Autodesk Fusion 360 part; units mm, degrees
sketch "Sketch1" plane through (0, 0, 0) normal (0, 0, 1) x (1, 0, 0)
  line L0 (66, 26) -> (-66, 26)
  line L1 (-70, 22) -> (-70, -22)
  line L2 (-66, -26) -> (66, -26)
  line L3 (70, -22) -> (70, 22)
  line L4 (70, 26) -> (-70, -26) construction
  line L5 (-70, 26) -> (70, -26) construction
  arc A0 (-70, -22) -> (-66, -26) centre (-66, -22) ccw
  arc A1 (-66, 26) -> (-70, 22) centre (-66, 22) ccw
  arc A2 (70, 22) -> (66, 26) centre (66, 22) ccw
  arc A3 (66, -26) -> (70, -22) centre (66, -22) ccw
  line L6 (-70, 26) -> (-57, 26) construction
  line L7 (-57, 26) -> (-57, 12.5) construction
  line L8 (-57, 12.5) -> (-70, 12.5) construction
  line L9 (-70, 12.5) -> (-70, 26) construction
  line L10 (70, 26) -> (57, 26) construction
  line L11 (57, 26) -> (57, 12.5) construction
  line L12 (57, 12.5) -> (70, 12.5) construction
  line L13 (70, 12.5) -> (70, 26) construction
  line L14 (-70, -26) -> (-57, -26) construction
  line L15 (-57, -26) -> (-57, -12.5) construction
  line L16 (-57, -12.5) -> (-70, -12.5) construction
  line L17 (-70, -12.5) -> (-70, -26) construction
  line L18 (70, -26) -> (57, -26) construction
  line L19 (57, -26) -> (57, -12.5) construction
  line L20 (57, -12.5) -> (70, -12.5) construction
  line L21 (70, -12.5) -> (70, -26) construction
  circle A4 centre (-57, 12.5) radius 2.2
  circle A5 centre (57, 12.5) radius 2.2
  circle A6 centre (-57, -12.5) radius 2.2
  circle A7 centre (57, -12.5) radius 2.2
  dimension "d1" = 140
  dimension "d2" = 52
  dimension "d3" = 4
  dimension "d4" = 13
  dimension "d5" = 13.5
  dimension "d6" = 13
  dimension "d7" = 13.5
  dimension "d8" = 13
  dimension "d9" = 13.5
  dimension "d10" = 13
  dimension "d11" = 13.5
  dimension "d12" = 4.4
  dimension "d13" = 4.4
  dimension "d14" = 4.4
  dimension "d15" = 4.4
extrude "Extrude1" add sketch "Sketch1" along normal blind 10
sketch "Sketch2" plane through (0, 0, 10) normal (0, 0, 1) x (-1, 0, 0)
  circle A0 centre (57, -12.5) radius 2.2
  circle A1 centre (-57, 12.5) radius 2.2
  circle A2 centre (57, 12.5) radius 2.2
  circle A3 centre (-57, -12.5) radius 2.2
  arc A4 (-66, 26) -> (-70, 22) centre (-66, 22) ccw
  line L0 (-70, 22) -> (-70, -22)
  arc A5 (-70, -22) -> (-66, -26) centre (-66, -22) ccw
  line L1 (-66, -26) -> (66, -26)
  arc A6 (66, -26) -> (70, -22) centre (66, -22) ccw
  line L2 (70, -22) -> (70, 22)
  arc A7 (70, 22) -> (66, 26) centre (66, 22) ccw
  line L3 (66, 26) -> (-66, 26)
  circle A8 centre (57, -12.5) radius 4
  circle A9 centre (57, 12.5) radius 4
  circle A10 centre (-57, -12.5) radius 4
  circle A11 centre (-57, 12.5) radius 4
  dimension "d18" = 8
  dimension "d19" = 8
  dimension "d20" = 8
  dimension "d21" = 8
extrude "Extrude2" cut sketch "Sketch2" against normal blind 4 contours A8 | A9 | A10 | A11
Work out the finished part from the listing and answer in its coordinate system (mm). A direction names the side the tool comes from. Give positions to 0.01 mm unless a question says otherwise; leave off trailing zeros. Loops run counter-clockwise (first coordinate to the right, second up) from the corner with the lowest first, then second, coordinate; pieces in that order, holes last. Notation, with made-up numbers: (11.5, 27.5) -> (23.5, 27.5) arc R32 cw to (23.5, 54.5) -> close; hole circle Ø4 at (85.5, 27.5). An arc over 180 degrees is marked (long way). One line per question, with ' | ' between items. Start each with the question number.
1) For faces 4 (the face through (70, 0, 5)), 5 (the face through (-59, -11, 6)), determine the directions among +Z, -Z, +X, -X, +Y, -Y from which every point of the face is accessible in a straight line to the end or side of a thin tool.
2) Section A-A, the plane x = 57 is taken. Determine the outline of the cut face in (y, z).
3) Section C-C, the plane z = 7.25 is taken. Determine the outline of the cut face in (x, y).
4) Each of these flat-tipped pins is pushed along its axis until it touches: pin 1 (6.5 mm diameter, centred on x = 57, y = -12.5, fed in from +Z); pin 2 (3.5 mm diameter, centred on x = 57, y = -12.5, fed in from +Z). Where does it stop, or does it pass through?
5) Section B-B, the plane y = -12.5 is taken. Determine the outline of the cut face in (x, z), then the cut area to 3 significant figures.
6) Determine the mould class of faces 1 (the face through (68.859, -24.797, 4.93)), 2 (the face through (55.38, -13.99, 2.96)), 3 (the face through (-1, 0, 0)) for opening direction X: +X half, -X half, draft (parallel to the pull), parting line (faces both ways), or undercut.
7) Straight lines are drawn through the part: L1, parallel to Y at x = -57, z = 1.75; L2, parallel to Y at x = -57, z = 8.6; L3, parallel to X at y = -11.5, z = 3.5. For each, find the intervals that lie inside material, in ascending order.
Resolved:
1) face 4: +Z, -Z, +X, +Y, -Y | face 5: +Z
2) outline: (-26, 0) -> (-14.7, 0) -> (-14.7, 6) -> (-16.5, 6) -> (-16.5, 10) -> (-26, 10) -> close; (-10.3, 0) -> (10.3, 0) -> (10.3, 6) -> (8.5, 6) -> (8.5, 10) -> (-8.5, 10) -> (-8.5, 6) -> (-10.3, 6) -> close; (14.7, 0) -> (26, 0) -> (26, 10) -> (16.5, 10) -> (16.5, 6) -> (14.7, 6) -> close
3) outline: (-70, -22) arc R4 ccw to (-66, -26) -> (66, -26) arc R4 ccw to (70, -22) -> (70, 22) arc R4 ccw to (66, 26) -> (-66, 26) arc R4 ccw to (-70, 22) -> close; hole circle Ø8 at (-57, -12.5); hole circle Ø8 at (-57, 12.5); hole circle Ø8 at (57, -12.5); hole circle Ø8 at (57, 12.5)
4) pin 1: z = 6 | pin 2: through
5) outline: (-70, 0) -> (-59.2, 0) -> (-59.2, 6) -> (-61, 6) -> (-61, 10) -> (-70, 10) -> close; (-54.8, 0) -> (54.8, 0) -> (54.8, 6) -> (53, 6) -> (53, 10) -> (-53, 10) -> (-53, 6) -> (-54.8, 6) -> close; (59.2, 0) -> (70, 0) -> (70, 10) -> (61, 10) -> (61, 6) -> (59.2, 6) -> close | area: 1,280 mm2
6) face 1: +X half | face 2: undercut | face 3: draft
7) L1: -26 to -14.7, -10.3 to 10.3, 14.7 to 26 | L2: -26 to -16.5, -8.5 to 8.5, 16.5 to 26 | L3: -70 to -58.96, -55.04 to 55.04, 58.96 to 70
